Work out the finished part from the listing and answer in its coordinate system (mm). A direction names the side the tool comes from. Give positions to 0.01 mm unless a question says otherwise; leave off trailing zeros. Order: outer loops, then holes, each group sorted by start corner. A loop starts at its lowest first (then second) coordinate and runs counter-clockwise, first axis right, second up. Notation, with made-up numbers: (79.25, 38.25) -> (109.25, 38.25) arc R10 ccw to (109.25, 55.25) -> close; hole circle Ø6 at (62, -29). An arc over 180 degrees is marked (long way). Answer as CSV lines item,"result". Start each with the question number.
1. A cutting plane is placed at A-A (x = 5.5). Give the vertices of the cut face in (y, z).
2. For faces 1 (the flat face through (0, 0, -3)), 2 (the flat face through (-5, -2, 2)), 3 (the flat face through (-3.68, -0.99, 1.74)), determine the directions among +Z, -Z, +X, -X, +Y, -Y from which every point of the face is accessible in a straight line to the end or side of a thin tool.
3. Find the intervals of material crossed by L1, parallel to Y at x = -2, z = 2; L2, parallel to Y at x = -3.25, z = 1; L3, parallel to Z at x = -1.5, y = -3.75, in increasing order.
4. For a pull along Z with two mould halves and no side action, classify faces 4 (the cylindrical face through (7.75, -0.54, 2.44)), 5 (the flat face through (16, 0, 0)), 6 (the flat face through (-3.679, -1.014, -1.724)) as released by +Z, released by -Z, zero draft, split by the parting line, or undercut.
5. Flat-ended cylindrical pins translate along their axes: pin 1 (1 mm diameter, centred on x = 7, z = 0, fed in from +Y); pin 2 (1.5 mm diameter, centred on x = 10.5, y = 3, fed in from -Z); pin 3 (1 mm diameter, centred on y = -2.5, z = 3.5, fed in from -X). Find the tip coordinate at first contact, or state that the pin passes through.
Autodesk Inventor part; units mm, degrees
ref_plane "Work Plane1" through (29, 0, 0) normal (0, -1, 0) x (1, 0, 0)
ref_plane "YZ Plane" through (0, 0, 0) normal (1, 0, 0) x (0, 1, 0)
ref_plane "XZ Plane" through (0, 0, 0) normal (0, 1, 0) x (-1, 0, 0)
sketch "Sketch1" plane through (0, 0, 0) normal (0, 0, 1) x (1, 0, 0)
  line L0 (-1.1667, 0) -> (16, 0)
  line L1 (16, 0) -> (16, 2.5)
  line L2 (16, 2.5) -> (0.8, 2.5)
  line L3 (0.8, 2.5) -> (0.3091, 2.5)
  line L4 (0.3091, 2.5) -> (0, 2.5)
  line L5 (0, 2.5) -> (0, 4.25)
  line L6 (0, 4.25) -> (-5, 4.25)
  line L7 (-5, 4.25) -> (-5, 2.3094)
  line L8 (-5, 2.3094) -> (-2.5, 2.3094)
  line L9 (-2.5, 2.3094) -> (-1.1667, 0)
  line L10 (-9.2, 0) -> (20.2, 0)
  line L11 (0, -0.85) -> (0, 5.1)
  line L12 (0.8, 2.5) -> (0, 2.5) construction
  dimension "d1" = 15.2
  dimension "d2" = 0.4909
  dimension "d3" = 5
  dimension "d4" = 2.5
  dimension "d5" = 60
  dimension "d6" = 5
  dimension "d7" = 5
  dimension "d8" = 4.6188
  dimension "d9" = 8.5
  dimension "d26" = 16
revolve "Body" add sketch "Sketch1" angle 360 about axis through (-1.1667, 0, 0) along (1, 0, 0)
sketch "Sketch2" plane through (-5, 0, 0) normal (-1, 0, 0) x (0, 0, 1)
  circle A0 centre (0, 0) radius 2.3094
  line L0 (0, -5.95) -> (0, 5.95)
  line L1 (-5.95, 0) -> (5.95, 0)
  line L2 (2.3094, 0) -> (1.1547, -2)
  line L3 (1.1547, -2) -> (-1.1547, -2)
  line L4 (-1.1547, -2) -> (-2.3094, 0)
  line L5 (-2.3094, 0) -> (-1.1547, 2)
  line L6 (-1.1547, 2) -> (1.1547, 2)
  line L7 (1.1547, 2) -> (2.3094, 0)
extrude "Slot" add sketch "Sketch2" against normal up to next contours L7 A0 | A0 L2 | L6 L0 A0 | A0 L0 L3 | L0 L6 A0 | A0 L3 L0 | L4 A0 | A0 L5
fillet "Fillet1" radius 0.5 1 edges at (-5, -4.25, 0)
thread "Thread"
chamfer "Chamfer1" distance 0.4908 distance2 0.4908 1 edges at (16, -2.5, 0) measured on face at (16, -1.1374, -1.1324)
ref_plane "Work Plane1" through (29, 0, 0) normal (0, -1, 0) x (1, 0, 0)
fillet "Fillet2" radius 0.2 1 edges at (0, -2.5, 0)
equation "\"d1\" = GEL"
equation "\"d3\" = KOH"
equation "\"d4\" = INTI"
equation "\"d6\" = GD"
equation "\"d7\" = BDM"
equation "\"d8\" = 1.1547 * SW"
equation "\"d9\" = KOD"
equation "\"d26\" = NLG"
equation "\"d30\" = R"
equation "\"d17\" = RR"
equation "\"d13\" = GEL"
equation "\"d15\" = -0.5 * SPD + 0.5 * GD"
equation "\"d16\" = GUL"
equation "\"GD\" = NND"
equation "\"NLG\" = 16"
equation "\"GEL\" = 15.2"
equation "\"KOD\" = 8.5"
equation "\"KOH\" = NND"
equation "\"INTI\" = 2.5"
equation "\"GAL\" = 0.61345 * PTC"
equation "\"GUL\" = 0.61345 * PTC"
equation "\"BDM\" = NND"
equation "\"SW\" = 4"
equation "\"RR\" = 0.5"
equation "\"SPD\" = NND - 1.2269 * PTC"
equation "\"R\" = 0.2"
equation "\"TOA\" = 30deg"
equation "\"GD1\" = THREADDIA - 1.2269 * PTC"
equation "\"THREADDIA\" = 5"
equation "\"FAWI\" = 45deg"
equation "\"PTC\" = 0.8"
equation "\"NND\" = 5"
equation "\"E0\" = 1.155 * SW"
properties part number "Screw GB/T 70.1 M5 x 16(1)" material "Steel, Mild"
Answer sheet:
1,outline,"circle Ø5 at (0, 0)"
2,face 1,"+X"
2,face 2,"+Z, -Z, -X, +Y, -Y"
2,face 3,"-X"
3,L1,"y = -3.75 to 3.75"
3,L2,"y = -4.13 to -2, 2 to 4.13"
3,L3,"z = -2 to 2"
4,face 4,"split by the parting line"
4,face 5,"zero draft"
4,face 6,"undercut"
5,pin 1,"stops at y = 2.5"
5,pin 2,"stops at z = -1.09"
5,pin 3,"stops at x = -5"
